Could you check a few things on this model? Use its own coordinates, in mm. A direction names the side the tool comes from. Give positions to 0.01 mm unless a question says otherwise; leave off trailing zeros. Loops run counter-clockwise (first coordinate to the right, second up) from the corner with the lowest first, then second, coordinate; pieces in that order, holes last. Notation, with made-up numbers: (-35.75, 77) - (21.25, 77) arc R27 ccw to (21.25, 106) - close; hole circle Ø6 at (-36, -1.5). An arc over 180 degrees is marked (long way). Answer in a Markdown table with one row per item. Add a question column.
```python
from build123d import *

# Parameters (mm, degrees)
SKETCH1_W           = 92.202
SKETCH1_H           = 35.56
BOSS_EXTRUDE3_DEPTH = 19.05
SKETCH4_W           = 83.82
SKETCH4_H           = 33.02
CUT_EXTRUDE1_DEPTH  = 12.7


with BuildPart() as part:
    # Sketch1 → Boss-Extrude3 (new body)
    with BuildSketch(Plane(origin=(0, 0, 0), x_dir=(1, 0, 0), z_dir=(0, 1, 0))):
        Polygon((-49.493351826, -85.725), (49.493351826, -85.725), (98.986703653, 0), (49.493351826, 85.725), (-49.493351826, 85.725), (-98.986703653, 0), align=None)
        with Locations((0.077086569, -103.505)):
            Rectangle(SKETCH1_W, SKETCH1_H)
    extrude(amount=BOSS_EXTRUDE3_DEPTH)

    # Sketch4 → Cut-Extrude1 (cut)
    with BuildSketch(Plane(origin=(0, 19.05, 0), x_dir=(1, 0, 0), z_dir=(0, 1, 0))):
        Polygon((46.011704472, -80.114854126), (92.387351129, -0.210122118), (46.375646657, 79.904732007), (-46.011704472, 80.114854126), (-92.387351129, 0.210122118), (-46.375646657, -79.904732007), align=None)
        with Locations((0.204587762, -96.425353803)):
            Rectangle(SKETCH4_W, SKETCH4_H)
    extrude(amount=-CUT_EXTRUDE1_DEPTH, mode=Mode.SUBTRACT)


solid = part.part
```
(1) I want a section at B-B on y = 2.75. Please give me the cut outline in (x, z) (3 decimals), then the cut area to 3 significant figures.
(2) I want a section at A-A on y = 13.25. Please give me the cut outline in (x, z) (3 decimals).
(3) We'd pull the mould along Z, two halves only. Please class faces 5 (the flat face through (74.59, 9.39, -42.26)), 6 (the flat face through (73.894, 9.392, 43.463)), 7 (the flat face through (-41.705, 13, 97)), 8 (the flat face through (66, 19.05, 48)): pulls with the +Z half, pulls with the -Z half, needs draft (parallel to the pull), parting line crosses it, or undercut.
(4) I want a section at D-D on x = 83. Please give me the cut outline in (y, z).
(5) For pin 1 Ø3 at (x, z) = (64.5, 19.5) entering from +Y; pin 2 Ø1.5 at (x, z) = (19.5, 33.5) entering from -Y; pin 3 Ø5.5 at (y, z) = (7, 106.5) entering from +X; pin 4 Ø10 at (y, z) = (12, 96) entering from -X, each with a flat end and sliding along its axis, tell me the tip position at first contact or that it passes through.
(6) On a 3-axis mill with a long thin cutter (end or side, diameter ignored), from which of +Z, -Z, +X, -X, +Y, -Y can I reach the whole of each face in a straight line? I mean faces 1 (the flat face through (-1, 9, 121.285)), 2 (the flat face through (-69.7, 12.79, 39.29)), 3 (the flat face through (46.178, 9, 104)), 4 (the flat face through (-46.024, 9, 104)). Say none if no direction works.
(7) I want a section at C-C on z = -22.5. Please give me the cut outline in (x, y), then the cut area to 3 significant figures.
(8) Please list where these lines run through material, in increasing order: line 1 (X direction, y = 9.75, z = 100.5); line 2 (Z direction, x = -29, y = 9.75) (3 decimals); line 3 (Y direction, x = 70, z = -13.5).
Reported:
| question | item | result |
|---|---|---|
| 1 | outline | (-98.987, 0) - (-49.493, -85.725) - (49.493, -85.725) - (98.987, 0) - (49.493, 85.725) - (46.178, 85.725) - (46.178, 121.285) - (-46.024, 121.285) - (-46.024, 85.725) - (-49.493, 85.725) - close |
| 1 | area | 28,700 mm² |
| 2 | outline | (-98.987, 0) - (-49.493, -85.725) - (49.493, -85.725) - (98.987, 0) - (49.493, 85.725) - (46.178, 85.725) - (46.178, 121.285) - (-46.024, 121.285) - (-46.024, 85.725) - (-49.493, 85.725) - close; hole (-92.387, -0.21) - (-46.012, -80.115) - (46.376, -79.905) - (92.387, 0.21) - (46.012, 80.115) - (42.115, 80.106) - (42.115, 112.935) - (-41.705, 112.935) - (-41.705, 79.915) - (-46.376, 79.905) - close |
| 3 | face 5 | pulls with the -Z half |
| 3 | face 6 | pulls with the +Z half |
| 3 | face 7 | undercut |
| 3 | face 8 | needs draft |
| 4 | outline | (0, -27.69) - (19.05, -27.69) - (19.05, -16.13) - (6.35, -16.13) - (6.35, 16.38) - (19.05, 16.38) - (19.05, 27.69) - (0, 27.69) - close |
| 5 | pin 1 | y = 6.35 |
| 5 | pin 2 | y = 0 |
| 5 | pin 3 | x = 46.18 |
| 5 | pin 4 | x = -46.02 |
| 6 | face 1 | +Z, +X, -X, +Y, -Y |
| 6 | face 2 | +Y |
| 6 | face 3 | +Z, +X, +Y, -Y |
| 6 | face 4 | +Z, -X, +Y, -Y |
| 7 | outline | (-86, 0) - (86, 0) - (86, 19.05) - (79.34, 19.05) - (79.34, 6.35) - (-79.45, 6.35) - (-79.45, 19.05) - (-86, 19.05) - close |
| 7 | area | 1,260 mm² |
| 8 | line 1 | -46.02 to -41.71, 42.11 to 46.18 |
| 8 | line 2 | -85.725 to -80.076, 112.935 to 121.285 |
| 8 | line 3 | 0 to 6.35 |
